Verification items for the finished model (mm, model axes). Face numbers are marked on the shaded views. A direction names the side the tool comes from. Round coordinates to 2 decimals unless told otherwise and drop trailing zeros. Order: outer loops, then holes, each group sorted by start corner. A loop starts at its lowest first (then second) coordinate and runs counter-clockwise, first axis right, second up. Notation, with made-up numbers: (24.25, 35.5) -> (29.25, 35.5) arc R3 cw to (29.25, 40.5) -> close; hole circle Ø3 at (34.5, -13). An arc over 180 degrees is marked (long way). Put each result on its own line as item: value.
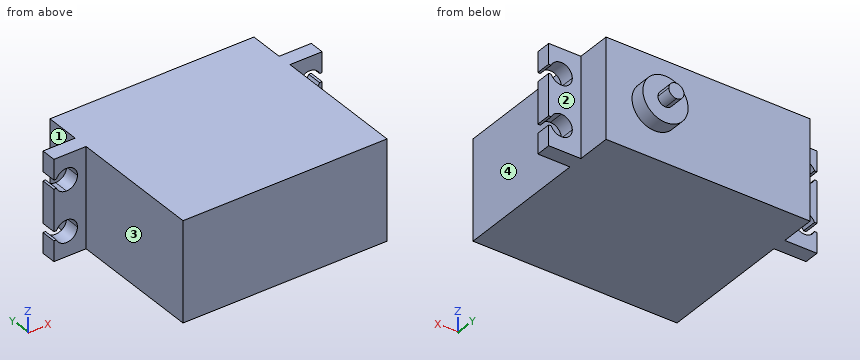
from build123d import *

# Parameters (mm, degrees)
ESQUISSE2_W        = 40.6
ESQUISSE2_H        = 19.82
BOSS_EXTRU_1_DEPTH = 36.6
BOSS_EXTRU_2_DEPTH = 6
BOSS_EXTRU_3_DEPTH = 3
ESQUISSE5_3_R      = 4.5
ESQUISSE5_3_R_2    = 1.5
BOSS_EXTRU_4_DEPTH = 3


with BuildPart() as part:
    # Esquisse2 → Boss.-Extru.1 (new body)
    with BuildSketch(Plane(origin=(0, 0, 0), x_dir=(1, 0, 0), z_dir=(0, 1, 0))):
        with Locations((-26.090639329, -15.529787325)):
            Rectangle(ESQUISSE2_W, ESQUISSE2_H)
    extrude(amount=BOSS_EXTRU_1_DEPTH)

    # Esquisse5 → Boss.-Extru.2 (add)
    with BuildSketch(Plane(origin=(0, 36.6, 0), x_dir=(1, 0, 0), z_dir=(0, 1, 0))):
        with BuildLine():
            ThreePointArc((-13.950639329, -15.529787325), (-14.389979157, -14.469127154), (-15.450639329, -14.029787325))
            Line((-15.450639329, -14.029787325), (-15.450639329, -17.029787325))
            ThreePointArc((-15.450639329, -17.029787325), (-14.389979157, -16.590447497), (-13.950639329, -15.529787325))
        make_face()
        with BuildLine():
            Line((-15.450639329, -17.029787325), (-15.450639329, -14.029787325))
            ThreePointArc((-15.450639329, -14.029787325), (-16.950639329, -15.529787325), (-15.450639329, -17.029787325))
        make_face()
    extrude(amount=BOSS_EXTRU_2_DEPTH)

    # Esquisse12 → Boss.-Extru.3 (add)
    with BuildSketch(Plane(origin=(0, 26.67, 0), x_dir=(-1, 0, 0), z_dir=(0, -1, 0))):
        with BuildLine():
            Line((52.293952717, -19.645007427), (52.790639329, -19.645007427))
            Line((52.790639329, -19.645007427), (52.790639329, -11.414567223))
            Line((52.790639329, -11.414567223), (52.293952717, -11.414567223))
            ThreePointArc((52.293952717, -11.414567223), (51.486137556, -12.364694404), (50.290639329, -12.719787325))
            Line((50.290639329, -12.719787325), (50.290639329, -18.339787325))
            ThreePointArc((50.290639329, -18.339787325), (51.486137556, -18.694880247), (52.293952717, -19.645007427))
        make_face()
        with BuildLine():
            Line((46.390639329, -10.529787325), (46.390639329, -20.529787325))
            Line((46.390639329, -20.529787325), (48.100639329, -20.529787325))
            ThreePointArc((48.100639329, -20.529787325), (48.742075478, -18.981223475), (50.290639329, -18.339787325))
            Line((50.290639329, -18.339787325), (50.290639329, -12.719787325))
            ThreePointArc((50.290639329, -12.719787325), (48.742075478, -12.078351176), (48.100639329, -10.529787325))
            Line((48.100639329, -10.529787325), (46.390639329, -10.529787325))
        make_face()
        with BuildLine():
            Line((46.390639329, -5.619787325), (46.390639329, -10.529787325))
            Line((46.390639329, -10.529787325), (48.100639329, -10.529787325))
            ThreePointArc((48.100639329, -10.529787325), (49.838508994, -8.386967184), (52.293952717, -9.645007427))
            Line((52.293952717, -9.645007427), (52.790639329, -9.645007427))
            Line((52.790639329, -9.645007427), (52.790639329, -5.619787325))
            Line((52.790639329, -5.619787325), (46.390639329, -5.619787325))
        make_face()
        with BuildLine():
            Line((46.390639329, -25.439787325), (52.790639329, -25.439787325))
            Line((52.790639329, -25.439787325), (52.790639329, -21.414567223))
            Line((52.790639329, -21.414567223), (52.293952717, -21.414567223))
            ThreePointArc((52.293952717, -21.414567223), (49.838508994, -22.672607467), (48.100639329, -20.529787325))
            Line((48.100639329, -20.529787325), (46.390639329, -20.529787325))
            Line((46.390639329, -20.529787325), (46.390639329, -25.439787325))
        make_face()
        with BuildLine():
            Line((4.080639329, -20.529787325), (5.790639329, -20.529787325))
            Line((5.790639329, -20.529787325), (5.790639329, -10.529787325))
            Line((5.790639329, -10.529787325), (4.080639329, -10.529787325))
            ThreePointArc((4.080639329, -10.529787325), (3.43920318, -12.078351176), (1.890639329, -12.719787325))
            Line((1.890639329, -12.719787325), (1.890639329, -18.339787325))
            ThreePointArc((1.890639329, -18.339787325), (3.43920318, -18.981223475), (4.080639329, -20.529787325))
        make_face()
        with BuildLine():
            ThreePointArc((-0.112674059, -19.645007427), (0.695141102, -18.694880247), (1.890639329, -18.339787325))
            Line((1.890639329, -18.339787325), (1.890639329, -12.719787325))
            ThreePointArc((1.890639329, -12.719787325), (0.695141102, -12.364694404), (-0.112674059, -11.414567223))
            Line((-0.112674059, -11.414567223), (-0.609360671, -11.414567223))
            Line((-0.609360671, -11.414567223), (-0.609360671, -19.645007427))
            Line((-0.609360671, -19.645007427), (-0.112674059, -19.645007427))
        make_face()
        with BuildLine():
            Line((5.790639329, -25.439787325), (5.790639329, -20.529787325))
            Line((5.790639329, -20.529787325), (4.080639329, -20.529787325))
            ThreePointArc((4.080639329, -20.529787325), (2.342769664, -22.672607467), (-0.112674059, -21.414567223))
            Line((-0.112674059, -21.414567223), (-0.609360671, -21.414567223))
            Line((-0.609360671, -21.414567223), (-0.609360671, -25.439787325))
            Line((-0.609360671, -25.439787325), (5.790639329, -25.439787325))
        make_face()
        with BuildLine():
            Line((4.080639329, -10.529787325), (5.790639329, -10.529787325))
            Line((5.790639329, -10.529787325), (5.790639329, -5.619787325))
            Line((5.790639329, -5.619787325), (-0.609360671, -5.619787325))
            Line((-0.609360671, -5.619787325), (-0.609360671, -9.645007427))
            Line((-0.609360671, -9.645007427), (-0.112674059, -9.645007427))
            ThreePointArc((-0.112674059, -9.645007427), (2.342769664, -8.386967184), (4.080639329, -10.529787325))
        make_face()
    extrude(amount=-BOSS_EXTRU_3_DEPTH)

    # Esquisse5_3 → Boss.-Extru.4 (add)
    with BuildSketch(Plane(origin=(0, 36.6, 0), x_dir=(1, 0, 0), z_dir=(0, 1, 0))):
        with Locations(Location((-15.450639329, -15.529787325, 0), (0, 0, 90))):
            Circle(ESQUISSE5_3_R)
        with Locations(Location((-15.450639329, -15.529787325, 0), (0, 0, 270))):
            Circle(ESQUISSE5_3_R_2, mode=Mode.SUBTRACT)
    extrude(amount=BOSS_EXTRU_4_DEPTH)


solid = part.part
Item 1: Material ranges on L1, parallel to Y at x = -26, z = 8.75; L2, parallel to X at y = 19, z = 18.25; L3, parallel to Y at x = -50, z = 7, recorded low to high. Write a range as [from, to].
Check sheet entries:
L1: y = [0, 36.6]
L2: x = [-46.39, -5.79]
L3: y = [26.67, 29.67]
Item 2: Section check B-B on x = -49. Record the boundary of the cut face in (y, z), then the cut area to 3 significant figures.
Check sheet entries:
outline: (26.67, 5.62) -> (29.67, 5.62) -> (29.67, 8.76) -> (26.67, 8.76) -> close; (26.67, 12.3) -> (29.67, 12.3) -> (29.67, 18.76) -> (26.67, 18.76) -> close; (26.67, 22.3) -> (29.67, 22.3) -> (29.67, 25.44) -> (26.67, 25.44) -> close
area: 38.2 mm^2
Item 3: Section check D-D on y = 39. Record the boundary of the cut face in (x, z).
Check sheet entries:
outline: circle Ø9 at (-15.45, 15.53)
Item 4: Section check C-C on x = -7. Record the boundary of the cut face in (y, z).
Check sheet entries:
outline: (0, 5.62) -> (36.6, 5.62) -> (36.6, 25.44) -> (0, 25.44) -> close
Item 5: Tool access check on the marked faces 1, 2, 3 and 4. Record the directions out of +Z, -Z, +X, -X, +Y, -Y that give a thin tool (end or side, any length) a straight path to the whole face; none if there is none.
Check sheet entries:
face 1: +Z, -Z, -X, +Y
face 2: +Z, -Z, +X, +Y
face 3: +Z, -Z, -X, -Y
face 4: +Z, -Z, +X, -Y
Item 6: Section check A-A on z = 12. Record the boundary of the cut face in (x, y), then the cut area to 3 significant figures.
Check sheet entries:
outline: (-52.79, 26.67) -> (-51.91, 26.67) -> (-51.91, 29.67) -> (-52.79, 29.67) -> close; (-48.67, 26.67) -> (-46.39, 26.67) -> (-46.39, 0) -> (-5.79, 0) -> (-5.79, 26.67) -> (-3.51, 26.67) -> (-3.51, 29.67) -> (-5.79, 29.67) -> (-5.79, 36.6) -> (-12.66, 36.6) -> (-12.66, 39.6) -> (-18.24, 39.6) -> (-18.24, 36.6) -> (-46.39, 36.6) -> (-46.39, 29.67) -> (-48.67, 29.67) -> close; (-0.27, 26.67) -> (0.61, 26.67) -> (0.61, 29.67) -> (-0.27, 29.67) -> close
area: 1,520 mm^2
Item 7: Gauge pin test, flat ends, axial feed: pin 1 Ø5 at (x, z) = (-2, 12) entering from +Y; pin 2 Ø2.5 at (x, z) = (-14, 16.5) entering from +Y; pin 3 Ø5 at (x, z) = (-20.5, 18.5) entering from +Y; pin 4 Ø7 at (x, z) = (-48.5, 18) entering from +Y. Record the tip position at first contact, or that the pin passes through.
Check sheet entries:
pin 1: stops at y = 29.67
pin 2: stops at y = 42.6
pin 3: stops at y = 39.6
pin 4: stops at y = 36.6
